Check sheet for the modelled part. Datum: model origin and axes. Units: mm. Give positions to 0.01 mm unless a question says otherwise; leave off trailing zeros. Write each loop counter-clockwise with the first axis right and the second up, starting at its lowest first coordinate (ties: lowest second). Pieces come first, ordered by that corner, then holes. Notation, with made-up numbers: M 0.5,-21.5 L 30.5,-21.5 A24 cw 30.5,-7.5 Z; hole C -20.75,88 d2. An arc over 180 degrees is marked long. Use CSV: the item, a comma, the result in double quotes. Start each with the question number.
1. Cross-section at B-B, the plane z = 0. Enter the section's corners in (x, y), and give its area (3 significant figures).
2. Mould release check, pull along X, two halves, no side actions. Record for faces 1 (the face through (47.69, 42.95, 15.02)), 2 (the face through (10.3, 44.11, -46.37)): +X half, -X half, draft (parallel to the pull), parting line (faces both ways), or undercut.
3. Scan lines: line 1 (Z direction, x = 0.5, y = 39); line 2 (Z direction, x = 42, y = 12); line 3 (X direction, y = 43.5, z = 1.5). Record each from-to range of solid material in increasing order.
4. Cross-section at C-C, the plane y = 76.5. Enter the section's corners in (x, z), and give its area (3 significant figures).
5. Cross-section at A-A, the plane x = 0. Enter the section's corners in (y, z).
6. Depth check by flat-ended pin: P1, Ø10, axis at y = 46.5, z = -37.5, coming from the +X side; P2, Ø2, axis at y = 41.5, z = -24.5, coming from the -X side; P3, Ø4, axis at y = 57.5, z = -8, coming from the -X side. Enter the tip coordinate at first touch or a pass-through.
from build123d import *

# Parameters (mm, degrees)
F0_R     = 50
F1_DEPTH = 87
F3_D     = 95
F3_DEPTH = 100
F3_TIP   = 28.5408794038


# Not quite as in the source:
# - a fillet or chamfer that OpenCascade refuses, or shapes differently, is made with other operations: its cross-section is extruded or revolved along the edge and cut away or added


with BuildPart() as f1:
    # F0 (on Front) → F1 (new body)
    with BuildSketch(Plane.XZ):
        Circle(F0_R)
    extrude(amount=-F1_DEPTH)

    # F3
    with Locations(Plane.XZ):
        with Locations((0, 0)):
            Hole(F3_D / 2, depth=F3_DEPTH)
            with Locations((0, 0, -(F3_DEPTH + F3_TIP / 2))):  # 118° drill point
                Cone(0, F3_D / 2, F3_TIP, mode=Mode.SUBTRACT)

    # F4: fillet of radius 5 on 2 edges, made by hand

    # F4_s1 → F4_t2 (revolve, cut)
    with BuildSketch(Plane.XY):
        with BuildLine():
            ThreePointArc((50, 4.3301270189), (49.3301270189, 1.8301270189), (47.5, 0))
            Line((47.5, 0), (50, 0))
            Line((50, 0), (50, 4.3301270189))
        make_face()
    revolve(axis=Axis((0, 0, 0), (0, -1, 0)), mode=Mode.SUBTRACT)

    # F4_s3 → F4_t4 (revolve, cut)
    with BuildSketch(Plane.XY):
        with BuildLine():
            ThreePointArc((50, 82.6698729811), (49.3301270189, 85.1698729811), (47.5, 87))
            Line((47.5, 87), (50, 87))
            Line((50, 87), (50, 82.6698729811))
        make_face()
    revolve(axis=Axis((0, 87, 0), (0, -1, 0)), mode=Mode.SUBTRACT)


solid = f1.part
Worked answers:
1,outline,"M -50,4.33 A5 ccw -47.5,0 L -47.5,87 A5 ccw -50,82.67 Z; M 47.5,0 A5 ccw 50,4.33 L 50,82.67 A5 ccw 47.5,87 Z"
1,area,"422 mm^2"
2,face 1,"parting line"
2,face 2,"undercut"
3,line 1,"z = -50 to -47.5, 47.5 to 50"
3,line 2,"z = -27.13 to -22.19, 22.19 to 27.13"
3,line 3,"x = -49.98 to -47.48, 47.48 to 49.98"
4,outline,"C 0,0 d100; hole C 0,0 d95"
4,area,"766 mm^2"
5,outline,"M 0,-47.5 A5 ccw 4.33,-50 L 82.67,-50 A5 ccw 87,-47.5 Z; M 0,47.5 L 87,47.5 A5 ccw 82.67,50 L 4.33,50 A5 ccw Z"
6,P1,"stops at x = 38"
6,P2,"stops at x = -44.13"
6,P3,"stops at x = -49.64"
